Input: part model. Units: mm. Frame: model coordinates. Round coordinates to 2 decimals unless told otherwise and drop trailing zeros. Loops run counter-clockwise (first coordinate to the right, second up) from the corner with the lowest first, then second, coordinate; pieces in that order, holes last.
(1) Cut plane B-B, the plane x = 8.53. Output: boundary loops of the cut face in (y, z).
(2) First-contact query: pin 1 Ø0.6 at (x, y) = (32.5, 1.5) entering from +Z; pin 2 Ø0.6 at (y, z) = (1, 25) entering from +X; pin 3 Ø1 at (x, y) = (35.5, 0.5) entering from -Z. Flat tips, straight axial feed; report the tip coordinate or a pass-through.
(3) Cut plane D-D, the plane z = 35. Output: boundary loops of the cut face in (x, y).
(4) Cut plane A-A, the plane z = 0. Output: boundary loops of the cut face in (x, y), and give its area (3 significant figures).
(5) Cut plane C-C, the plane x = -45. Output: boundary loops of the cut face in (y, z).
(6) Line query: line 1 (Z direction, x = 30.5, y = 1.05); line 2 (Z direction, x = 54, y = 0.7); line 3 (Z direction, x = -54, y = 0.75). Output: solid intervals per line, ascending.
(7) Draft query along X for faces 1 (the face through (1, 0, 1)), 2 (the face through (-69.994, 0.986, 0.93)), 3 (the face through (2.527, 0.986, -34.775)), 4 (the face through (23.26, 0.986, -20.483)). Return one class per face: released by +X, released by -X, zero draft, split by the parting line, or undercut.
Autodesk Inventor part; units mm, degrees
ref_plane "YZ Plane" through (0, 0, 0) normal (1, 0, 0) x (0, 1, 0)
ref_plane "XZ Plane" through (0, 0, 0) normal (0, 1, 0) x (-1, 0, 0)
ref_plane "XY Plane" through (0, 0, 0) normal (0, 0, 1) x (1, 0, 0)
sketch "Esboço1" plane through (0, 0, 0) normal (0, 1, 0) x (-1, 0, 0)
  arc A0 (-40.7914, 56.8864) -> (-40.7914, -56.8864) centre (0, 0) ccw
  arc A1 (40.7914, -56.8864) -> (40.7914, 56.8864) centre (0, 0) ccw
  line L0 (-11.73, 29.4903) -> (42.27, 29.4903) construction
  line L1 (42.27, 29.4903) -> (42.27, -38.5097) construction
  line L2 (42.27, -38.5097) -> (-11.73, -38.5097) construction
  line L3 (-11.73, -38.5097) -> (-11.73, 29.4903) construction
  line L4 (-19, 28) -> (-44, 28)
  line L5 (-44, 28) -> (-44, 24)
  line L6 (-44, 24) -> (-19, 24)
  line L7 (-19, 24) -> (-19, 28)
  line L8 (-19, -24) -> (-44, -24)
  line L9 (-44, -24) -> (-44, -28)
  line L10 (-44, -28) -> (-19, -28)
  line L11 (-19, -28) -> (-19, -24)
  circle A2 centre (39.73, 14.2503) radius 2
  circle A3 centre (24.49, -36.5497) radius 2
  circle A4 centre (-3.45, -36.5497) radius 2
  circle A5 centre (54, -22) radius 2
  circle A6 centre (54, 22) radius 2
  circle A7 centre (-54, 22) radius 2
  circle A8 centre (-54, -22) radius 2
  line L12 (0, 45) -> (-38, 45)
  line L13 (-40, 47) -> (-40, 56.4801)
  line L14 (0, 45) -> (38, 45)
  line L15 (40, 47) -> (40, 56.4801)
  line L16 (0, -45) -> (-38, -45)
  line L17 (-40, -47) -> (-40, -56.4801)
  line L18 (0, -45) -> (38, -45)
  line L19 (40, -47) -> (40, -56.4801)
  arc A9 (40.7914, -56.8864) -> (40.7914, 56.8864) centre (0, 0) ccw
  arc A10 (-40.7914, 56.8864) -> (-40.7914, -56.8864) centre (0, 0) ccw
  circle A11 centre (-8.53, 15.2503) radius 2
  circle A12 centre (-23, -18.5) radius 2
  circle A13 centre (-23, 18.5) radius 2
  arc A14 (38, 45) -> (40, 47) centre (38, 47) ccw
  arc A15 (-40, 47) -> (-38, 45) centre (-38, 47) ccw
  arc A16 (-38, -45) -> (-40, -47) centre (-38, -47) ccw
  arc A17 (40, -47) -> (38, -45) centre (38, -47) ccw
  arc A18 (40, -56.4801) -> (40.7914, -56.8864) centre (40.5, -56.4801) ccw
  arc A19 (40.7914, 56.8864) -> (40, 56.4801) centre (40.5, 56.4801) ccw
  arc A20 (-40, 56.4801) -> (-40.7914, 56.8864) centre (-40.5, 56.4801) ccw
  arc A21 (-40.7914, -56.8864) -> (-40, -56.4801) centre (-40.5, -56.4801) ccw
  line L20 (-27.75, 32.5) -> (-27.75, 38.5)
  line L21 (-27.75, 32.5) -> (-27.25, 32.5)
  line L22 (-27, 38.5) -> (-27.75, 38.5)
  line L23 (-33, 38.5) -> (-34, 38.5)
  line L24 (-34, 38.5) -> (-34, 32.5)
  line L25 (-34, 32.5) -> (-33, 32.5)
  line L26 (-33, 32.5) -> (-33, 38.5)
  line L27 (-27.75, 38.5) -> (-26.75, 38.5)
  line L28 (-26.75, 38.5) -> (-26.75, 32.5)
  line L29 (-26.75, 32.5) -> (-27.75, 32.5)
  line L30 (-27.75, 32.5) -> (-27.75, 38.5)
  circle A22 centre (45, -40) radius 2
  circle A23 centre (45, 40) radius 2
  circle A24 centre (54, 0) radius 2
  point P0 (-40, 45)
  point P1 (40, 45)
  point P2 (-40, -45)
  point P3 (40, -45)
  dimension "d144" = 0.5
extrude "Extrusão3" add sketch "Esboço1" along normal blind 2
properties part number "base 1" material "Plástico PC/ABS"
Reported:
1. outline: (0, -45) - (2, -45) - (2, 13.25) - (0, 13.25) - close; (0, 17.25) - (2, 17.25) - (2, 45) - (0, 45) - close
2. pin 1: stops at z = 45
2. pin 2: stops at x = 65.5
2. pin 3: stops at z = -45
3. outline: (-60.62, 0) - (26.75, 0) - (26.75, 2) - (-60.62, 2) - close; (27.75, 0) - (33, 0) - (33, 2) - (27.75, 2) - close; (34, 0) - (60.62, 0) - (60.62, 2) - (34, 2) - close
4. outline: (-70, 0) - (-56, 0) - (-56, 2) - (-70, 2) - close; (-52, 0) - (70, 0) - (70, 2) - (-52, 2) - close
4. area: 272 mm2
5. outline: (0, -53.62) - (2, -53.62) - (2, -42) - (0, -42) - close; (0, -38) - (2, -38) - (2, 38) - (0, 38) - close; (0, 42) - (2, 42) - (2, 53.62) - (0, 53.62) - close
6. line 1: z = -45 to -28, -24 to 24, 28 to 45
6. line 2: z = -44.54 to -24, -20 to 20, 24 to 44.54
6. line 3: z = -44.54 to -24, -20 to -2, 2 to 20, 24 to 44.54
7. face 1: zero draft
7. face 2: released by -X
7. face 3: undercut
7. face 4: undercut
